CAD build for the part. Positions are in the model's coordinates, mm. Round coordinates to 2 decimals unless told otherwise and drop trailing zeros. Loops run counter-clockwise (first coordinate to the right, second up) from the corner with the lowest first, then second, coordinate; pieces in that order, holes last. Notation, with made-up numbers: (-35, 1.5) - (21, 1.5) arc R24 ccw to (21, 35.5) - close; hole circle Ø11 at (-11, 10.5). An arc over 180 degrees is marked (long way). Use one line per item in the form item = value.
from build123d import *

# Parameters (mm, degrees)
F0_R     = 11.2
F1_DEPTH = 7


# Not quite as in the source:
# - ends of sketch curves that miss each other by under 0.0002 mm in the source are joined


with BuildPart() as f1:
    # F0 (on Top) → F1 (new body)
    with BuildSketch(Plane.XY):
        with BuildLine():
            ThreePointArc((24.885011592, 0), (13.8227560246, 6.7091569655), (10.5100821241, 19.2156543591))
            ThreePointArc((10.5100821241, 19.2156543591), (13.1664242497, 28.1426673783), (9.267685926, 36.601246125))
            Line((9.267685926, 36.601246125), (0, 50.6668537855))
            Line((0, 50.6668537855), (-10.6134602306, 35.0499921165))
            Line((-10.6134602306, 35.0499921165), (-11.2040059959, 34.1810510431))
            ThreePointArc((-11.2040059959, 34.1810510431), (-13.1594893438, 28.235141726), (-12.1560699163, 22.0568812763))
            ThreePointArc((-12.1560699163, 22.0568812763), (-12.4352425028, 9.122108449), (-21.6098500078, 0))
            ThreePointArc((-21.6098500078, 0), (-30.6478922927, -2.1487015261), (-36.0320947169, -9.7191574841))
            Line((-36.0320947169, -9.7191574841), (-43.5794253076, -24.7780127605))
            Line((-43.5794253076, -24.7780127605), (-25.4962357758, -26.1061598733))
            ThreePointArc((-25.4962357758, -26.1061598733), (-18.4080870059, -25.3666213531), (-12.7374420281, -21.0500769317))
            ThreePointArc((-12.7374420281, -21.0500769317), (-1.3959205219, -14.82446107), (11.0913608835, -18.2088500145))
            ThreePointArc((11.0913608835, -18.2088500145), (17.4993705689, -24.9467054642), (26.7596797789, -25.7881075822))
            ThreePointArc((26.7596797789, -25.7881075822), (35.0805283727, -18.9135515404), (35.4898237471, -8.127981579))
            ThreePointArc((35.4898237471, -8.127981579), (31.3336966338, -2.63072231), (24.9734656325, 0.0227120051))
            Line((24.9734656325, 0.0227120051), (24.885011592, 0))
        make_face()
        with Locations((-23.2474307999, -13.063953107)):
            Circle(F0_R, mode=Mode.SUBTRACT)
        with Locations((23.2474307999, -13.063953107)):
            Circle(F0_R, mode=Mode.SUBTRACT)
        Circle(F0_R, mode=Mode.SUBTRACT)
        with Locations((0, 27.2017781838)):
            Circle(F0_R, mode=Mode.SUBTRACT)
        with BuildLine():
            Line((43.5474583602, -24.7964688862), (35.4898237471, -8.127981579))
            ThreePointArc((35.4898237471, -8.127981579), (35.0805283727, -18.9135515404), (26.7596797789, -25.7881075822))
            Line((26.7596797789, -25.7881075822), (43.5474583602, -24.7964688862))
        make_face()
    extrude(amount=F1_DEPTH)


solid = f1.part
1) Slice it at C-C (z = 2.75). Write the cut outline in (x, y).
Report:
outline = (-43.58, -24.78) - (-25.5, -26.11) arc R13.2 ccw to (-12.74, -21.05) arc R17.3 cw to (11.09, -18.21) arc R13.2 ccw to (26.76, -25.79) - (43.55, -24.8) - (35.49, -8.13) arc R13.2 ccw to (24.97, 0.02) - (24.89, 0) arc R17.3 cw to (10.51, 19.22) arc R13.2 ccw to (9.27, 36.6) - (0, 50.67) - (-11.2, 34.18) arc R13.2 ccw to (-12.16, 22.06) arc R17.3 cw to (-21.61, 0) arc R13.2 ccw to (-36.03, -9.72) - close; hole circle Ø22.4 at (-23.25, -13.06); hole circle Ø22.4 at (0, 0); hole circle Ø22.4 at (0, 27.2); hole circle Ø22.4 at (23.25, -13.06)
2) Flat gauge pins, fed straight in: pin 1 (1.5 mm diameter, centred on y = 21.5, z = 5.5, fed in from +X); pin 2 (4 mm diameter, centred on y = -0.5, z = 2.5, fed in from +X); pin 3 (2 mm diameter, centred on y = -11, z = 4, fed in from -X). Where does each tip first touch, or does it go through?
Report:
pin_1 = 12.24
pin_2 = 31.16
pin_3 = -37.18
3) Drill centre lines: probe 1 along Y at (x, z) = (-23, 2.5); probe 2 along Y at (x, z) = (-8, 0.75); probe 3 along X at (y, z) = (-9.5, 1.25). Where is each one in solid material? Low to high.
Report:
probe_1 = -26.29 to -24.26, -1.87 to 0.1
probe_2 = -17.02 to -7.84, 7.84 to 19.36, 35.04 to 38.9
probe_3 = -35.97 to -33.87, -12.63 to -5.93, 5.93 to 12.63, 33.87 to 36.15
4) Slice it at A-A (x = -15). Write the cut outline in (y, z).
Report:
outline = (-23.38, 0) - (-20.64, 0) - (-20.64, 7) - (-23.38, 7) - close; (-5.49, 0) - (4.92, 0) - (4.92, 7) - (-5.49, 7) - close
5) Two-plate mould, pull along Y, no slides. Class faces 1 (the flat face through (-39.75, -17.14, 3.45)), 2 (the cylindrical face through (-12.363, 9.293, 3.451)), 3 (the flat face through (35, -25.3, 3.5)), 4 (the cylindrical face through (-13.152, 28.323, 3.451)): +Y half, -Y half, draft (parallel to the pull), parting line (faces both ways), or undercut.
Report:
face_1 = +Y half
face_2 = undercut
face_3 = -Y half
face_4 = undercut
6) Slice it at B-B (y = 23.5). Write the cut outline in (x, z).
Report:
outline = (-12.67, 0) - (-10.57, 0) - (-10.57, 7) - (-12.67, 7) - close; (10.57, 0) - (12.67, 0) - (12.67, 7) - (10.57, 7) - close
